Input: dimensioned drawing with shaded views. Units: mm. Origin: part minimum x, y, z. Round coordinates to 2 decimals unless told otherwise and drop trailing zeros. Loops run counter-clockwise (first coordinate to the right, second up) from the corner with the lowest first, then second, coordinate; pieces in that order, holes last. Notation, with made-up numbers: (11, -26) - (64, -26) arc R25 ccw to (64, -12) - close; hole circle Ø1 at (89, -37). An arc over 180 degrees is marked (long way). One line per question, with ' | ' between items. Start each with the question number.
1. Ray query, line 1 (Y direction, x = 48.5, z = 0.25); line 2 (X direction, y = 31, z = 1.65); line 3 (X direction, y = 12.5, z = 1.35). Return the intervals inside material, ascending.
2. Cut plane B-B (z = 2.55). Return loops of the section in (x, y).
3. Pin query (flat end, axial travel): pin 1 (1.5 mm diameter, centred on x = 40, z = 1, fed in from +Y); pin 2 (0.9 mm diameter, centred on y = 45.5, z = 1.5, fed in from -X). Return the tip coordinate at first contact, or that it passes through.
4. Cut plane A-A (x = 24). Return loops of the section in (y, z), then the cut area to 3 significant figures.
5. Cut plane C-C (y = 41). Return loops of the section in (x, z), then the cut area to 3 significant figures.
6. Cut plane D-D (x = 81.5). Return loops of the section in (y, z).
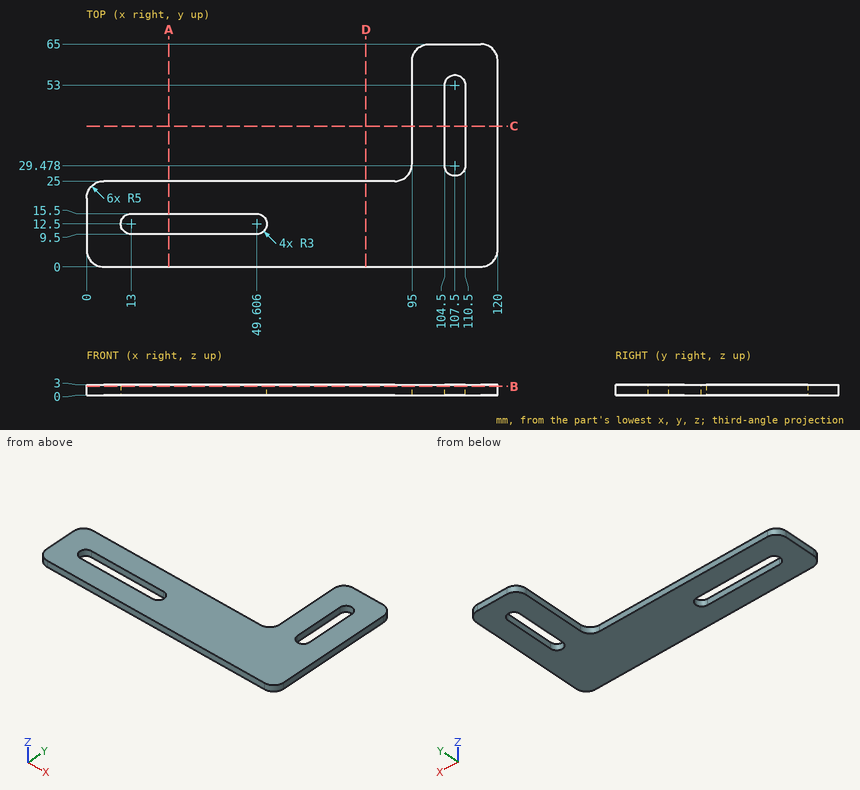
Answers follow:
1) line 1: y = 0 to 9.5, 15.5 to 25 | line 2: x = 95 to 104.5, 110.5 to 120 | line 3: x = 0 to 10, 52.61 to 120
2) outline: (0, 5) arc R5 ccw to (5, 0) - (115, 0) arc R5 ccw to (120, 5) - (120, 60) arc R5 ccw to (115, 65) - (100, 65) arc R5 ccw to (95, 60) - (95, 30) arc R5 cw to (90, 25) - (5, 25) arc R5 ccw to (0, 20) - close; hole (13, 9.5) - (49.61, 9.5) arc R3 ccw to (49.61, 15.5) - (13, 15.5) arc R3 ccw to start; hole (104.5, 29.48) arc R3 ccw to (110.5, 29.48) - (110.5, 53) arc R3 ccw to (104.5, 53) - close
3) pin 1: stops at y = 25 | pin 2: stops at x = 95
4) outline: (0, 0) - (9.5, 0) - (9.5, 3) - (0, 3) - close; (15.5, 0) - (25, 0) - (25, 3) - (15.5, 3) - close | area: 57.0 mm2
5) outline: (95, 0) - (104.5, 0) - (104.5, 3) - (95, 3) - close; (110.5, 0) - (120, 0) - (120, 3) - (110.5, 3) - close | area: 57.0 mm2
6) outline: (0, 0) - (25, 0) - (25, 3) - (0, 3) - close
